```python
from build123d import *

# Parameters (mm, degrees)
F0_W     = 84.6
F0_H     = 70
F1_DEPTH = 6.3
F2_DEPTH = 6.3
F3_W     = 80.6
F3_H     = 10.6
F4_DEPTH = 69
F6_DEPTH = 25
F7_W     = 10
F7_H     = 40
F8_DEPTH = 5


# Not quite as in the source:
# - ends of sketch curves that miss each other by under 0.0002 mm in the source are joined


with BuildPart() as f1:
    # F0 (on Front) → F1 (new body)
    with BuildSketch(Plane.XZ):
        Rectangle(F0_W, F0_H)
    extrude(amount=F1_DEPTH)

    # F0 (on Front) → F2 (join)
    with BuildSketch(Plane.XZ):
        Rectangle(F0_W, F0_H)
    extrude(amount=-F2_DEPTH)

    # F3 (on face) → F4 (cut)
    with BuildSketch(Plane.XY.offset(35)):
        Rectangle(F3_W, F3_H)
    extrude(amount=-F4_DEPTH, mode=Mode.SUBTRACT)

    # F5 (on face) → F6 (cut)
    with BuildSketch(Plane.XZ.offset(6.3)):
        Polygon((-30, 30), (-30, -30), (30, -30), (30, 30), (30.0000030547, 35), (-30, 35), align=None)
    extrude(amount=-F6_DEPTH, mode=Mode.SUBTRACT)

    # F7 (on face) → F8 (join)
    with BuildSketch(Plane(origin=(0, 0, -35), x_dir=(1, 0, 0), z_dir=(0, 0, -1))):
        with Locations((-37.3, 0)):
            Rectangle(F7_W, F7_H)
        with Locations((37.3, 0)):
            Rectangle(F7_W, F7_H)
    extrude(amount=F8_DEPTH)


solid = f1.part
```
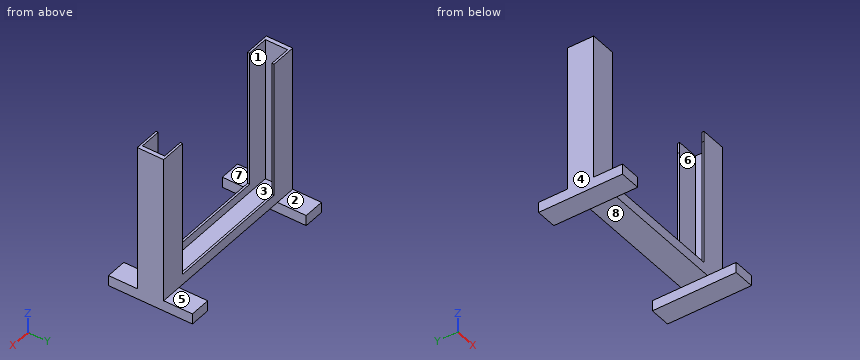
Geometry: final body of the model. Coordinates: model frame, mm. Face numbers are marked on the shaded views. A direction names the side the tool comes from. Give positions to 0.01 mm unless a question says otherwise; leave off trailing zeros. Loops run counter-clockwise (first coordinate to the right, second up) from the corner with the lowest first, then second, coordinate; pieces in that order, holes last. Notation, with made-up numbers: (-4, -39) -> (14, -39) arc R36 cw to (14, -3) -> close; hole circle Ø9 at (-4.5, 78.25). An arc over 180 degrees is marked (long way). Return JSON: item names as keys, results as strings.
Item 1: Section B-B, the plane y = -15. Output: boundary loops of the cut face in (x, z).
Filled in:
{"outline": "(-42.3, -40) -> (-32.3, -40) -> (-32.3, -35) -> (-42.3, -35) -> close; (32.3, -40) -> (42.3, -40) -> (42.3, -35) -> (32.3, -35) -> close"}
Item 2: Line query: line 1 (Y direction, x = -32, z = 1); line 2 (X direction, y = 5.5, z = 28.5); line 3 (X direction, y = -9.5, z = -35.5). Output: solid intervals per line, ascending.
Filled in:
{"line 1": "-6.3 to -5.3, 5.3 to 6.3", "line 2": "-42.3 to -30, 30 to 42.3", "line 3": "-42.3 to -32.3, 32.3 to 42.3"}
Item 3: Section D-D, the plane x = 1. Output: boundary loops of the cut face in (y, z).
Filled in:
{"outline": "(-6.3, -35) -> (6.3, -35) -> (6.3, -30) -> (5.3, -30) -> (5.3, -34) -> (-5.3, -34) -> (-5.3, -30) -> (-6.3, -30) -> close"}
Item 4: Section C-C, the plane y = -0.5. Output: boundary loops of the cut face in (x, z), plus the area to 3 significant figures.
Filled in:
{"outline": "(-42.3, -40) -> (-32.3, -40) -> (-32.3, -35) -> (32.3, -35) -> (32.3, -40) -> (42.3, -40) -> (42.3, 35) -> (40.3, 35) -> (40.3, -34) -> (-40.3, -34) -> (-40.3, 35) -> (-42.3, 35) -> close", "area": "461 mm^2"}
Item 5: Mould query, pull axis X, two halves, no side actions, for the marked faces 1, 2, 3 and 4. Classes: released by +X, released by -X, zero draft, split by the parting line, or undercut.
Filled in:
{"face 1": "undercut", "face 2": "zero draft", "face 3": "undercut", "face 4": "released by -X"}
Item 6: Section A-A, the plane z = 24. Output: boundary loops of the cut face in (x, y).
Filled in:
{"outline": "(-42.3, -6.3) -> (-30, -6.3) -> (-30, -5.3) -> (-40.3, -5.3) -> (-40.3, 5.3) -> (-30, 5.3) -> (-30, 6.3) -> (-42.3, 6.3) -> close; (30, -6.3) -> (42.3, -6.3) -> (42.3, 6.3) -> (30, 6.3) -> (30, 5.3) -> (40.3, 5.3) -> (40.3, -5.3) -> (30, -5.3) -> close"}
Item 7: Access query for the marked faces 5, 6, 7 and 8. Directions: +Z, -Z, +X, -X, +Y, -Y. A direction counts if a zero-diameter tool reaches every point of the face in a straight line with its end or side. Return the directions, or none.
Filled in:
{"face 5": "+Z, +X, -X, +Y", "face 6": "+Z", "face 7": "+Z, +X, -X, -Y", "face 8": "-Z, +Y, -Y"}
Item 8: Pin query (flat end, axial travel): P1, Ø0.8, axis at x = -2, y = -5.5, coming from the +Z side; P2, Ø4, axis at x = 32.5, z = 22.5, coming from the -Y side; P3, Ø8, axis at x = 36.5, y = 10.5, coming from the +Z side; P4, Ø10, axis at y = -14.5, z = -14.5, coming from the +X side. Return the tip coordinate at first contact, or that it passes through.
Filled in:
{"P1": "z = -30", "P2": "y = -6.3", "P3": "z = -35", "P4": "through"}
